Read the model definition and answer for the solid it produces. Units are mm, in the model's axes. Face numbers are marked on the shaded views. A direction names the side the tool comes from. Round coordinates to 2 decimals unless told otherwise and drop trailing zeros. Loops run counter-clockwise (first coordinate to the right, second up) from the corner with the lowest first, then second, coordinate; pieces in that order, holes last. Notation, with made-up numbers: (-18, 53.5) - (8, 53.5) arc R19 ccw to (8, 80.5) - close; hole circle Ø4 at (1.5, 79.5). An arc over 180 degrees is marked (long way). Use CSV: the item, a comma, the result in double quotes. Start each with the question number.
1. Consider line 1 along Z through (x, y) = (-1.75, -2.1); line 2 along X through (y, z) = (-3.85, 9); line 3 along Z through (x, y) = (3.25, -2.5). Determine where each line is inside the solid, lowest interval first.
2. Given pin 1 Ø5 at (x, z) = (1.63, 24.21) entering from +Y; pin 2 Ø3 at (x, z) = (-5.37, 10.21) entering from -Y; pin 3 Ø5 at (x, z) = (-1.87, 6.71) entering from -Y, each flat-ended and moving along its own axis, determine where each tip first touches the part or whether it passes through.
3. Find section A-A (x = -8.25). Give the vertices of the cut face in (y, z).
4. Find section C-C (y = -2.45). State how many separate pieces and enclosed holes the cut face has, and give its area (3 significant figures).
5. A tool of negligible diameter and unlimited length cuts with its end or side. For the marked faces 1, 2 and 3, from which of +Z, -Z, +X, -X, +Y, -Y can it reach the whole face along a straight path? Write none if from no direction.
6. Find section D-D (x = 5.5). Give the vertices of the cut face in (y, z).
7. Find section B-B (z = 21.75). Give the vertices of the cut face in (x, y).
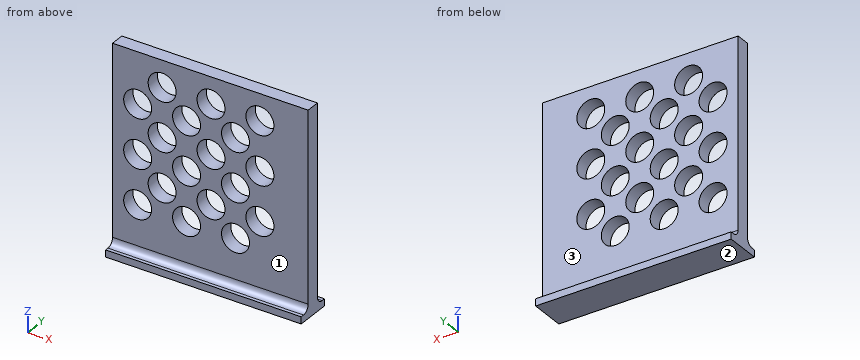
Autodesk Inventor part; units mm, degrees
ref_plane "YZ Plane" through (0, 0, 0) normal (1, 0, 0) x (0, 1, 0)
ref_plane "XZ Plane" through (0, 0, 0) normal (0, 1, 0) x (-1, 0, 0)
ref_plane "XY Plane" through (0, 0, 0) normal (0, 0, 1) x (1, 0, 0)
sketch "Sketch1" plane through (0, 0, 0) normal (0, 0, 1) x (1, 0, 0)
  line L0 (-19.4684, -0.3877) -> (8.5316, -0.3877)
  line L1 (8.5316, -0.3877) -> (8.5316, -5.3877)
  line L2 (8.5316, -5.3877) -> (-19.4684, -5.3877)
  line L3 (-19.4684, -5.3877) -> (-19.4684, -0.3877)
  line L4 (-19.4684, -1.8877) -> (8.5316, -1.8877)
  line L5 (8.5316, -1.8877) -> (8.5316, -3.8877)
  line L6 (8.5316, -3.8877) -> (-19.4684, -3.8877)
  line L7 (-19.4684, -3.8877) -> (-19.4684, -1.8877)
  point P0 (0, 0)
  dimension "d0" = 28
  dimension "d1" = 5
  dimension "d4" = 2
  dimension "d5" = 28
  dimension "d7" = 1.5
  dimension "d56" = 0
extrude "Extrusion1" add sketch "Sketch1" along normal blind 28 contours L4 L1 L6 L3
extrude "Extrusion2" add sketch "Sketch1" against normal blind 1
fillet "Fillet1" radius 1 2 edges at (-5.4684, -3.8877, 0) (-5.4684, -1.8877, 0)
sketch "Sketch2" plane through (-19.4684, -3.8877, 28) normal (0, -1, 0) x (1, 0, 0)
  line L0 (27, -1) -> (1, -1)
  line L1 (1, -1) -> (1, -17)
  line L2 (1, -17) -> (27, -17)
  line L3 (27, -17) -> (27, -1)
  line L4 (0, 0) -> (28, 0)
  line L5 (2.3536, -1) -> (7.3536, -1) construction
  line L6 (8.0711, -1) -> (5.2426, -3.8284)
  line L7 (5.2426, -3.8284) -> (2.4142, -1)
  line L8 (1, -2.4142) -> (3.8284, -5.2426)
  line L9 (3.8284, -5.2426) -> (1, -8.0711)
  line L10 (1, -8.0711) -> (2.4142, -9.4853)
  line L11 (2.4142, -9.4853) -> (5.2426, -6.6569)
  line L12 (5.2426, -6.6569) -> (8.0711, -9.4853)
  line L13 (8.0711, -9.4853) -> (9.4853, -8.0711)
  line L14 (9.4853, -8.0711) -> (6.6569, -5.2426)
  line L15 (6.6569, -5.2426) -> (9.4853, -2.4142)
  line L16 (9.4853, -2.4142) -> (8.0711, -1)
  line L17 (2.4142, -1) -> (1, -2.4142)
  line L18 (9.4853, -2.4142) -> (9.4853, -8.0711)
  line L19 (8.0711, -9.4853) -> (2.4142, -9.4853)
  line L20 (1, -8.0711) -> (1, -2.4142)
  line L21 (2.4142, -1) -> (8.0711, -1)
  line L22 (28, -27) -> (28, 0)
  line L23 (0, -27) -> (0, 0)
  point P0 (19.4684, -28)
  dimension "d28" = 4
  dimension "d29" = 2
  dimension "d30" = 4
  dimension "d31" = 2
  dimension "d32" = 4
  dimension "d39" = 8.4853
  dimension "d40" = 1
  dimension "d41" = 1
  dimension "d42" = 1
extrude "Extrusion3" [suppressed]
pattern_linear "Rectangular Pattern1" [suppressed]
sketch "Sketch3" plane through (-19.4684, -3.8877, 28) normal (0, -1, 0) x (1, 0, 0)
  line L0 (3, -3) -> (3, -21) construction
  line L1 (2, -3) -> (2, -21)
  line L2 (4, -21) -> (4, -3)
  arc A0 (4, -3) -> (2, -3) centre (3, -3) ccw
  arc A1 (2, -21) -> (4, -21) centre (3, -21) ccw
  line L3 (0, 0) -> (28, 0)
  line L4 (0, -27) -> (0, 0)
  point P0 (19.4684, -28)
  point P1 (3, -12)
  dimension "d43" = 2
  dimension "d44" = 3
  dimension "d45" = 18
  dimension "d48" = 3
extrude "Extrusion4" [suppressed]
pattern_linear "Rectangular Pattern2" [suppressed]
fillet "Fillet2" [suppressed]
sketch "Sketch4" plane through (-19.4684, -3.8877, 28) normal (0, -1, 0) x (1, 0, 0)
  line L0 (0, -27) -> (0, 0)
  circle A0 centre (3.5936, -7.288) radius 2
  circle A1 centre (7.0936, -3.788) radius 2
  point P0 (19.4684, -28)
  dimension "d80" = 4
  dimension "d81" = 4
  dimension "d82" = 3.5
  dimension "d83" = 3.5
extrude "Extrusion5" cut sketch "Sketch4" against normal blind 10
pattern_linear "Rectangular Pattern3" count 3 spacing 7 along (1, 0, 0) count 3 spacing 7 along (0, 0, -1) of "Extrusion5"
equation "\"d0\" = d5"
equation "\"d28\" = d32"
equation "\"d29\" = d31"
equation "\"d30\" = d32"
equation "\"d80\" = d81"
equation "\"d83\" = d82"
properties part number "vent test circle"
Filled sheet:
1,line 1,"z = -1 to 4.72, 8.71 to 11.72, 15.71 to 18.72, 22.71 to 28"
1,line 2,"x = -19.47 to -13.97, -10.78 to -6.97, -3.78 to 0.03, 3.22 to 8.53"
1,line 3,"z = -1 to 9.05, 11.38 to 16.05, 18.38 to 23.05, 25.38 to 28"
2,pin 1,"stops at y = -1.89"
2,pin 2,"passes through"
2,pin 3,"stops at y = -3.89"
3,outline,"(-5.39, -1) - (-0.39, -1) - (-0.39, 0) - (-0.89, 0) arc R1 cw to (-1.89, 1) - (-1.89, 4.81) - (-3.89, 4.81) - (-3.89, 1) arc R1 cw to (-4.89, 0) - (-5.39, 0) - close; (-3.89, 8.61) - (-1.89, 8.61) - (-1.89, 11.81) - (-3.89, 11.81) - close; (-3.89, 15.61) - (-1.89, 15.61) - (-1.89, 18.81) - (-3.89, 18.81) - close; (-3.89, 22.61) - (-1.89, 22.61) - (-1.89, 28) - (-3.89, 28) - close"
4,separate pieces,"1"
4,enclosed holes,"18"
4,area,"586 mm²"
5,face 1,"+Z, +X, -X, -Y"
5,face 2,"-Z, +X, -X, +Y, -Y"
5,face 3,"+Z, +X, -X, +Y"
6,outline,"(-5.39, -1) - (-0.39, -1) - (-0.39, 0) - (-0.89, 0) arc R1 cw to (-1.89, 1) - (-1.89, 28) - (-3.89, 28) - (-3.89, 1) arc R1 cw to (-4.89, 0) - (-5.39, 0) - close"
7,outline,"(-19.47, -3.89) - (-17.58, -3.89) - (-17.58, -1.89) - (-19.47, -1.89) - close; (-14.17, -3.89) - (-10.58, -3.89) - (-10.58, -1.89) - (-14.17, -1.89) - close; (-7.17, -3.89) - (-3.58, -3.89) - (-3.58, -1.89) - (-7.17, -1.89) - close; (-0.17, -3.89) - (8.53, -3.89) - (8.53, -1.89) - (-0.17, -1.89) - close"
